The listing builds one solid part. Answer for the finished solid, in the listing's coordinates (mm). A direction names the side the tool comes from. Round coordinates to 2 decimals unless told otherwise and drop trailing zeros. Loops run counter-clockwise (first coordinate to the right, second up) from the corner with the lowest first, then second, coordinate; pieces in that order, holes last. Notation, with made-up numbers: (17, -30.75) -> (62, -30.75) arc R11 ccw to (62, -24.75) -> close; hole circle Ø11 at (-39.5, 83.25). An arc over 180 degrees is marked (long way). Write each question's results on one line, items separated by ' | '. Start each with the question number.
(1) Straight lines are drawn through the part: probe 1 along Y at (x, z) = (0, 2.5); probe 2 along Y at (x, z) = (16, 0); probe 3 along Z at (x, y) = (-8, 31.5). For each, find the intervals that lie inside material, in ascending order.
(2) Determine the mould class of faces 1 (the face through (0, 16, 7)), 2 (the face through (-1.08, 27.12, -0.07)), 3 (the face through (6.76, 12, 21.46)) for opening direction X: released by +X, released by -X, zero draft, split by the parting line, or undercut.
(3) The part is cut by section C-C (y = 5). Determine the outline of the cut face in (x, z).
(4) For faces 4 (the face through (0, 15, 13)), 5 (the face through (-9.43, 27.4, -4.4)), 6 (the face through (9.43, 27.6, 4.4)), determine the directions among +Z, -Z, +X, -X, +Y, -Y from which every point of the face is accessible in a straight line to the end or side of a thin tool.
(5) The part is cut by section A-A (y = 32). Determine the outline of the cut face in (x, z), plus the area to 3 significant figures.
(6) Flat-ended cylindrical pins translate along their axes: pin 1 (3 mm diameter, centred on x = -19, z = 5, fed in from +Y); pin 2 (12 mm diameter, centred on x = 16.5, z = -5.5, fed in from +Y); pin 3 (1.8 mm diameter, centred on y = 30, z = 0.5, fed in from +X). Find the tip coordinate at first contact, or state that the pin passes through.
(7) The part is cut by section B-B (y = 25). Determine the outline of the cut face in (x, z), plus the area to 3 significant figures.
```python
from build123d import *

# Parameters (mm, degrees)
SKETCH1_R           = 25
BOSS_EXTRUDE1_DEPTH = 10
SKETCH2_R           = 22.5
BOSS_EXTRUDE2_DEPTH = 5
FILLET3_R           = 5
FILLET4_R           = 2
FILLET5_R           = 2
SKETCH3_R           = 5
BOSS_EXTRUDE3_DEPTH = 5
FILLET6_R           = 2
FILLET7_R           = 2
FILLET8_R           = 5


with BuildPart() as part:
    # Sketch1 → Boss-Extrude1 (new body)
    with BuildSketch(Plane(origin=(0, 0, 0), x_dir=(1, 0, 0), z_dir=(0, 1, 0))):
        with Locations(Location((0, 0, 0), (0, 0, 270))):
            Circle(SKETCH1_R)
    extrude(amount=BOSS_EXTRUDE1_DEPTH)

    # Sketch2 → Boss-Extrude2 (add)
    with BuildSketch(Plane(origin=(0, 10, 0), x_dir=(1, 0, 0), z_dir=(0, 1, 0))):
        with Locations(Location((0, 0, 0), (0, 0, 270))):
            Circle(SKETCH2_R)
    extrude(amount=BOSS_EXTRUDE2_DEPTH)

    # Fillet3
    # the kernel refuses this fillet: 5 mm, written as the material it takes off along each edge
    with BuildSketch(Plane(origin=(0, 10, 0), x_dir=(0, 0, 1), z_dir=(-1, 0, 0))) as fillet3_piece_1:
        with BuildLine():
            CenterArc((20, -4.330127019), FILLET3_R, 0, 60)
            Line((22.5, 0), (22.55, 0.08660254))
            ThreePointArc((22.55, 0.08660254), (23.75, 0.1), (25, 0.1))
            Line((25, 0.1), (25.1, 0))
            Line((25.1, 0), (25.1, -4.330127019))
            Line((25.1, -4.330127019), (25, -4.330127019))
        make_face()
    revolve(axis=Axis((0, 10, 0), (0, 1, 0)), mode=Mode.SUBTRACT)

    # Fillet4
    fillet4_edges = [part.edges().sort_by_distance(p)[0] for p in [
        (0, 15, -22.5),
    ]]
    fillet(fillet4_edges, radius=FILLET4_R)

    # Fillet5
    fillet5_edges = [part.edges().sort_by_distance(p)[0] for p in [
        (0, 10, -22.5),
    ]]
    fillet(fillet5_edges, radius=FILLET5_R)

    # Sketch3 → Boss-Extrude3 (add, symmetric)
    with BuildSketch(Plane.XY):
        with BuildLine():
            Line((-10, 15), (10, 15))
            Line((10, 15), (10, 35))
            ThreePointArc((10, 35), (8.535533906, 38.535533906), (5, 40))
            Line((5, 40), (-5, 40))
            ThreePointArc((-5, 40), (-8.535533906, 38.535533906), (-10, 35))
            Line((-10, 35), (-10, 15))
        make_face()
        with Locations((0, 32)):
            Circle(SKETCH3_R, mode=Mode.SUBTRACT)
    extrude(amount=BOSS_EXTRUDE3_DEPTH, both=True)

    # Fillet6
    fillet6_edges = [part.edges().sort_by_distance(p)[0] for p in [
        (-10, 25, 5),
        (10, 25, 5),
        (8.535533906, 38.535533906, 5),
        (0, 40, 5),
        (-8.535533906, 38.535533906, 5),
    ]]
    fillet(fillet6_edges, radius=FILLET6_R)

    # Fillet7
    fillet7_edges = [part.edges().sort_by_distance(p)[0] for p in [
        (-10, 25, -5),
        (-8.535533906, 38.535533906, -5),
        (0, 40, -5),
        (8.535533906, 38.535533906, -5),
        (10, 25, -5),
    ]]
    fillet(fillet7_edges, radius=FILLET7_R)

    # Fillet8
    fillet8_edges = [part.edges().sort_by_distance(p)[0] for p in [
        (0, 15, 5),
        (9.414213562, 15, 4.414213562),
        (-9.414213562, 15, 4.414213562),
        (10, 15, 0),
        (0, 15, -5),
        (-10, 15, 0),
        (9.414213562, 15, -4.414213562),
        (-9.414213562, 15, -4.414213562),
    ]]
    fillet(fillet8_edges, radius=FILLET8_R)


solid = part.part
```
Checked values:
1) probe 1: y = 0 to 27, 37 to 40 | probe 2: y = 0 to 15 | probe 3: z = -5 to 5
2) face 1: zero draft | face 2: undercut | face 3: split by the parting line
3) outline: circle Ø50 at (0, 0)
4) face 4: +Y | face 5: -Z, -X, +Y | face 6: +Z, +X, +Y
5) outline: (-10, -3) arc R2 ccw to (-8, -5) -> (-5, -5) -> (-5, 5) -> (-8, 5) arc R2 ccw to (-10, 3) -> close; (5, -5) -> (8, -5) arc R2 ccw to (10, -3) -> (10, 3) arc R2 ccw to (8, 5) -> (5, 5) -> close | area: 96.6 mm2
6) pin 1: stops at y = 15 | pin 2: stops at y = 17.2 | pin 3: stops at x = 10
7) outline: (-10, -3) arc R2 ccw to (-8, -5) -> (8, -5) arc R2 ccw to (10, -3) -> (10, 3) arc R2 ccw to (8, 5) -> (-8, 5) arc R2 ccw to (-10, 3) -> close | area: 197 mm2
